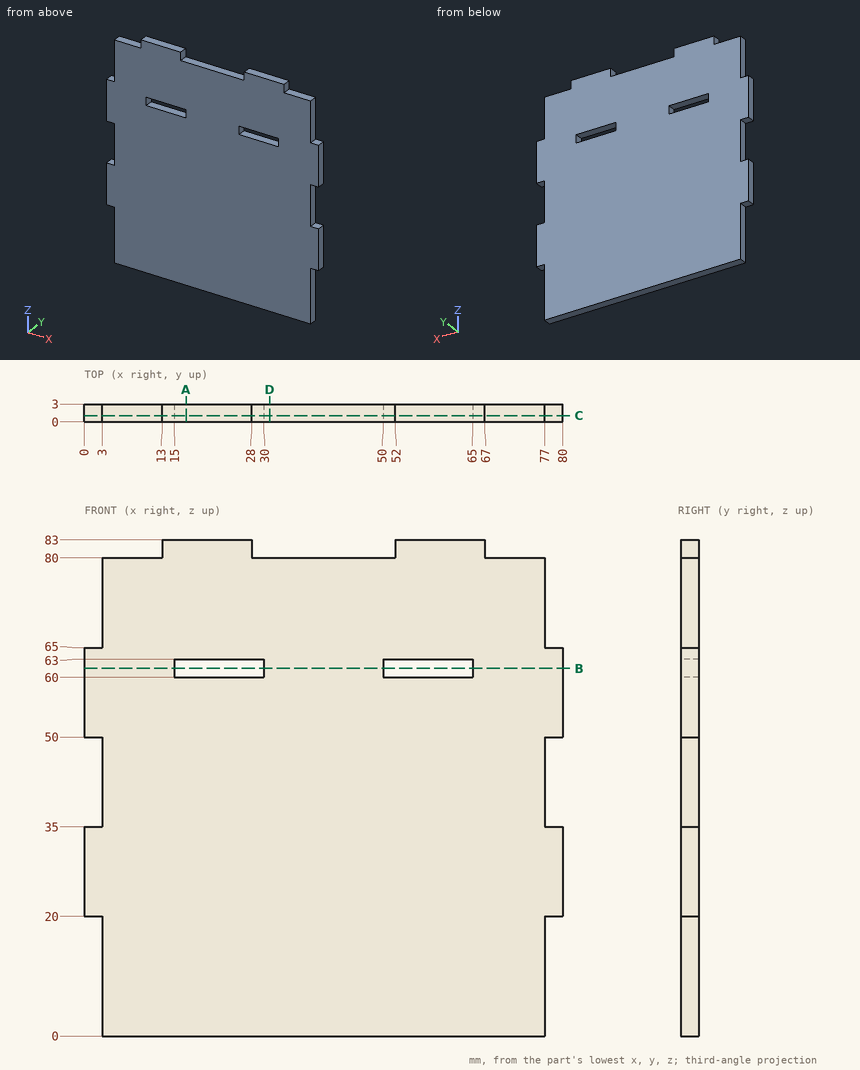
Verification items for this drawing (mm, ordinates from the low corner). Coordinates: 2 decimals unless noted, no trailing zeros. Order: outer loops, then holes, each group sorted by start corner. A loop starts at its lowest first (then second) coordinate and runs counter-clockwise, first axis right, second up. Notation, with made-up numbers: (50, -13.5) -> (59, -13.5) arc R31 cw to (59, 22.5) -> close; hole circle Ø5 at (40.5, 40). An arc over 180 degrees is marked (long way). Answer as CSV lines item,"result". Start each with the question number.
1) Gauge pin test, flat ends, axial feed: pin 1 Ø0.9 at (x, y) = (78.5, 1.5) entering from +Z; pin 2 Ø0.9 at (y, z) = (2, 81.5) entering from -X; pin 3 Ø3 at (x, z) = (35, 25) entering from -Y; pin 4 Ø0.9 at (x, y) = (71.5, 1) entering from +Z. Record the tip position at first contact, or that the pin passes through.
2) Material ranges on L1, parallel to Z at x = 25.5, y = 0.8; L2, parallel to Z at x = 68.5, y = 1.05; L3, parallel to X at y = 0.9, z = 16.5, recorded low to high. Write a range as [from, to].
3) Cross-section at B-B, the plane z = 61.5. Record the boundary of the cut face in (x, y), then the cut area to 3 significant figures.
4) Cross-section at C-C, the plane y = 1.05. Give the number of separate pieces and of enclosed holes in the cut face, then the cut area to 3 significant figures.
5) Cross-section at D-D, the plane x = 31. Record the boundary of the cut face in (y, z).
6) Cross-section at A-A, the plane x = 17. Record the boundary of the cut face in (y, z), then the cut area to 3 significant figures.
Conclusion:
1,pin 1,"stops at z = 65"
1,pin 2,"stops at x = 13"
1,pin 3,"stops at y = 0"
1,pin 4,"stops at z = 80"
2,L1,"z = [0, 60], [63, 83]"
2,L2,"z = [0, 80]"
2,L3,"x = [3, 77]"
3,outline,"(0, 0) -> (15, 0) -> (15, 3) -> (0, 3) -> close; (30, 0) -> (50, 0) -> (50, 3) -> (30, 3) -> close; (65, 0) -> (80, 0) -> (80, 3) -> (65, 3) -> close"
3,area,"150 mm²"
4,separate pieces,"1"
4,enclosed holes,"2"
4,area,"6,100 mm²"
5,outline,"(0, 0) -> (3, 0) -> (3, 80) -> (0, 80) -> close"
6,outline,"(0, 0) -> (3, 0) -> (3, 60) -> (0, 60) -> close; (0, 63) -> (3, 63) -> (3, 83) -> (0, 83) -> close"
6,area,"240 mm²"
